```python
from build123d import *

# Parameters (mm, degrees)
SKETCH_1_W          = 31
SKETCH_1_H          = 38
EXTRUDE_1_DEPTH     = 40.75
SKETCH_2_W          = 8
SKETCH_2_H          = 16.5
CUT_EXTRUDE_1_DEPTH = 40.75
SKETCH_3_W          = 25
SKETCH_3_H          = 34.75
CUT_EXTRUDE_2_DEPTH = 34.5
SKETCH_4_R          = 12.5
CUT_EXTRUDE_3_DEPTH = 34.5
SKETCH_5_R          = 1.6
EXTRUDE_2_DEPTH     = 3
EXTRUDE_5_DEPTH     = 5
SKETCH_9_R          = 1.7
CUT_EXTRUDE_4_DEPTH = 10
SKETCH_11_R         = 1.7
CUT_EXTRUDE_5_DEPTH = 10
SKETCH_12_W         = 31
SKETCH_12_H         = 16.5
CUT_EXTRUDE_6_DEPTH = 8


with BuildPart() as part:
    # 草图1 → 凸台-拉伸1 (new body)
    with BuildSketch(Plane.XY):
        with Locations((15.5, 19)):
            Rectangle(SKETCH_1_W, SKETCH_1_H)
    extrude(amount=-EXTRUDE_1_DEPTH)

    # 草图2 → 切除-拉伸1 (cut)
    with BuildSketch(Plane(origin=(31, 0, 0), x_dir=(0, 0, -1), z_dir=(1, 0, 0))):
        with Locations((36.75, 29.75)):
            Rectangle(SKETCH_2_W, SKETCH_2_H)
    extrude(amount=-CUT_EXTRUDE_1_DEPTH, mode=Mode.SUBTRACT)

    # 草图3 → 切除-拉伸2 (cut)
    with BuildSketch(Plane(origin=(0, 38, 0), x_dir=(1, 0, 0), z_dir=(0, 1, 0))):
        with Locations((15.5, 20.375)):
            Rectangle(SKETCH_3_W, SKETCH_3_H)
    extrude(amount=-CUT_EXTRUDE_2_DEPTH, mode=Mode.SUBTRACT)

    # 草图4 → 切除-拉伸3 (cut)
    with BuildSketch(Plane.XY):
        with Locations((15.5, 38)):
            Circle(SKETCH_4_R)
    extrude(amount=-CUT_EXTRUDE_3_DEPTH, mode=Mode.SUBTRACT)

    # 草图5 → 凸台-拉伸2 (add)
    with BuildSketch(Plane(origin=(0, 38, 0), x_dir=(1, 0, 0), z_dir=(0, 1, 0))):
        with BuildLine():
            Line((36, 23.375), (31, 23.375))
            Line((31, 23.375), (31, 17.375))
            Line((31, 17.375), (36, 17.375))
            ThreePointArc((36, 17.375), (39, 20.375), (36, 23.375))
        make_face()
        with Locations((36, 20.375)):
            Circle(SKETCH_5_R, mode=Mode.SUBTRACT)
        with BuildLine():
            Line((0, 23.375), (0, 17.375))
            Line((0, 17.375), (-5, 17.375))
            ThreePointArc((-5, 17.375), (-8, 20.375), (-5, 23.375))
            Line((-5, 23.375), (0, 23.375))
        make_face()
        with Locations((-5, 20.375)):
            Circle(SKETCH_5_R, mode=Mode.SUBTRACT)
    extrude(amount=-EXTRUDE_2_DEPTH)

    # 草图8 → 凸台-拉伸5 (add)
    with BuildSketch(Plane.XZ):
        with BuildLine():
            Line((-20.766160191, -40.75), (51.766160191, -40.75))
            ThreePointArc((51.766160191, -40.75), (15.5, 16.125), (-20.766160191, -40.75))
        make_face()
    extrude(amount=-EXTRUDE_5_DEPTH)

    # 草图9 → 切除-拉伸4 (cut)
    with BuildSketch(Plane(origin=(0, 5, 0), x_dir=(1, 0, 0), z_dir=(0, 1, 0))):
        with Locations((40, 8.875)):
            Circle(SKETCH_9_R)
        with Locations((-9, 8.875)):
            Circle(SKETCH_9_R)
    extrude(amount=-CUT_EXTRUDE_4_DEPTH, mode=Mode.SUBTRACT)

    # 草图11 → 切除-拉伸5 (cut)
    with BuildSketch(Plane(origin=(0, 5, 0), x_dir=(1, 0, 0), z_dir=(0, 1, 0))):
        with Locations((15.5, -8.125)):
            Circle(SKETCH_11_R)
    extrude(amount=-CUT_EXTRUDE_5_DEPTH, mode=Mode.SUBTRACT)

    # 草图12 → 切除-拉伸6 (cut)
    with BuildSketch(Plane.XY):
        with Locations((15.5, 29.75)):
            Rectangle(SKETCH_12_W, SKETCH_12_H)
    extrude(amount=-CUT_EXTRUDE_6_DEPTH, mode=Mode.SUBTRACT)


solid = part.part
```
The listing builds one solid part. Answer for the finished solid, in the listing's coordinates (mm). A direction names the side the tool comes from. Coordinates: 2 decimals unless noted, no trailing zeros. Write each loop counter-clockwise with the first axis right and the second up, starting at its lowest first coordinate (ties: lowest second). Pieces come first, ordered by that corner, then holes. Notation, with made-up numbers: (-35, 80) -> (3, 80) arc R22 ccw to (3, 118) -> close; hole circle Ø11 at (71.5, 28). An arc over 180 degrees is marked (long way). Write each question's results on one line, items separated by ' | '. Start each with the question number.
1) A cutting plane is placed at A-A (y = 24). Determine the outline of the cut face in (x, z), then the cut area to 4 significant figures.
2) A cutting plane is placed at D-D (z = -26). Determine the outline of the cut face in (x, y).
3) A cutting plane is placed at B-B (y = 10.5). Determine the outline of the cut face in (x, z), then the cut area to 4 significant figures.
4) Flat-ended cylindrical pins translate along their axes: pin 1 Ø12 at (y, z) = (25.5, -27) entering from +X; pin 2 Ø6 at (y, z) = (12.5, 4) entering from +X; pin 3 Ø16.5 at (y, z) = (28, -20) entering from +X; pin 4 Ø0.9 at (x, y) = (2, 29) entering from -Z. Find the tip coordinate at first contact, or state that the pin passes through.
5) A cutting plane is placed at C-C (x = -9). Determine the outline of the cut face in (y, z) (3 decimals), then the cut area to 3 significant figures.
6) For a pull along Y with two mould halves and no side action, classify faces 1 (the flat face through (-3, 35, -20)), 2 (the flat face through (15, 0, -18)), 3 (the flat face through (15, 8, -40.75)) as +Y half, -Y half, draft (parallel to the pull), parting line (faces both ways), or undercut.
7) A tool of negligible diameter and unlimited length cuts with its end or side. For faces 4 (the flat face through (16, 21.5, -38)), 5 (the flat face through (1, 30, -8)), 6 (the flat face through (34, 37, -23.375)), 7 (the flat face through (33, 37, -17.375)), 8 (the cylindrical face through (34.821, 36.521, -21.456)), from which of +Z, -Z, +X, -X, +Y, -Y can it reach the whole face along a straight path? Write none if from no direction.
8) Straight lines are drawn through the part: probe 1 along Z at (x, y) = (-5, 37.05) (3 decimals); probe 2 along X at (y, z) = (9.5, -17); probe 3 along Z at (x, y) = (13.5, 11). For each, find the intervals that lie inside material, in ascending order.
Values follow:
1) outline: (0, -32.75) -> (3, -32.75) -> (3, -8) -> (0, -8) -> close; (28, -32.75) -> (31, -32.75) -> (31, -8) -> (28, -8) -> close | area: 148.5 mm²
2) outline: (-24.44, 0) -> (55.44, 0) -> (55.44, 5) -> (31, 5) -> (31, 38) -> (28, 38) -> (28, 5) -> (3, 5) -> (3, 38) -> (0, 38) -> (0, 5) -> (-24.44, 5) -> close
3) outline: (0, -40.75) -> (31, -40.75) -> (31, 0) -> (0, 0) -> close; hole (3, -37.75) -> (28, -37.75) -> (28, -3) -> (3, -3) -> close | area: 394.5 mm²
4) pin 1: x = 31 | pin 2: through | pin 3: x = 39 | pin 4: z = -32.75
5) outline: (0, -40.75) -> (5, -40.75) -> (5, -10.575) -> (0, -10.575) -> close; (0, -7.175) -> (5, -7.175) -> (5, 7.744) -> (0, 7.744) -> close | area: 225 mm²
6) face 1: undercut | face 2: -Y half | face 3: draft
7) face 4: -Z, +X, -X, +Y | face 5: +Z, +X, -X, +Y | face 6: -Z, +X, +Y | face 7: +Z, +X, +Y | face 8: +Y
8) probe 1: -23.375 to -21.975, -18.775 to -17.375 | probe 2: 0 to 3, 28 to 31 | probe 3: -40.75 to -37.75, -3 to 0
